```python
from build123d import *

# Parameters (mm, degrees)
SKETCH1_W           = 12.7
SKETCH1_H           = 12.7
BOSS_EXTRUDE1_DEPTH = 1.6002
SKETCH2_W           = 12.7
SKETCH2_H           = 11.7602
BOSS_EXTRUDE2_DEPTH = 1.6002
SKETCH3_W           = 12.7
SKETCH3_H           = 1.6002
BOSS_EXTRUDE3_DEPTH = 9.525
SKETCH4_R           = 2.5527
CUT_EXTRUDE1_DEPTH  = 22.187985158
FILLET1_R           = 0.762


with BuildPart() as part:
    # Sketch1 → Boss-Extrude1 (new body)
    with BuildSketch(Plane(origin=(0, 0, 0), x_dir=(1, 0, 0), z_dir=(0, 1, 0))):
        Rectangle(SKETCH1_W, SKETCH1_H)
    extrude(amount=BOSS_EXTRUDE1_DEPTH)

    # Sketch2 → Boss-Extrude2 (add)
    with BuildSketch(Plane(origin=(6.35, 0, 0), x_dir=(0, 0, -1), z_dir=(1, 0, 0))):
        with Locations((0, -4.2799)):
            Rectangle(SKETCH2_W, SKETCH2_H)
    boss_extrude2 = extrude(amount=BOSS_EXTRUDE2_DEPTH)

    # Sketch3 → Boss-Extrude3 (add)
    with BuildSketch(Plane(origin=(7.9502, 0, 0), x_dir=(0, 0, -1), z_dir=(1, 0, 0))):
        with Locations((0, -9.3599)):
            Rectangle(SKETCH3_W, SKETCH3_H)
    boss_extrude3 = extrude(amount=BOSS_EXTRUDE3_DEPTH)

    # Sketch4 → Cut-Extrude1 (cut, through all)
    with BuildSketch(Plane(origin=(0, -8.5598, 0), x_dir=(1, 0, 0), z_dir=(0, 1, 0))):
        with Locations(Location((12.7127, 0, 0), (0, 0, 270))):
            Circle(SKETCH4_R)
    cut_extrude1 = extrude(amount=-CUT_EXTRUDE1_DEPTH, mode=Mode.SUBTRACT)

    # Mirror2: Boss-Extrude2, Boss-Extrude3, Cut-Extrude1 across plane
    add(boss_extrude2.mirror(Plane(origin=(0, 0, 0), x_dir=(0, 0, 1), z_dir=(1, 0, 0))))
    add(boss_extrude3.mirror(Plane(origin=(0, 0, 0), x_dir=(0, 0, 1), z_dir=(1, 0, 0))))
    add(cut_extrude1.mirror(Plane(origin=(0, 0, 0), x_dir=(0, 0, 1), z_dir=(1, 0, 0))), mode=Mode.SUBTRACT)

    # Fillet1
    fillet1_edges = [part.edges().sort_by_distance(p)[0] for p in [
        (6.35, -10.16, 0),
        (-6.35, -10.16, 0),
        (6.35, 0, 0),
        (-6.35, 0, 0),
        (-7.9502, -8.5598, 0),
        (-7.9502, 1.6002, 0),
        (7.9502, 1.6002, 0),
        (7.9502, -8.5598, 0),
    ]]
    fillet(fillet1_edges, radius=FILLET1_R)


solid = part.part
```
Geometry check sheet. Reference: the model listing, model coordinates, mm. A direction names the side the tool comes from. Coordinates: 2 decimals unless noted, no trailing zeros. Loops run counter-clockwise (first coordinate to the right, second up) from the corner with the lowest first, then second, coordinate; pieces in that order, holes last.
Item 1: Access from +Z, -Z, +X, -X, +Y, -Y to the whole of each face (thin tool, end or side, straight path). Record for faces 5 (the face through (-7.95, -3, 0)), 6 (the face through (6.35, -5, 0)), 7 (the face through (7.95, -3, 0)).
Item 2: Sectioned sample at C-C, the plane x = -14. Record the boundary of the cut face in (y, z), then the cut area to 3 significant figures.
Item 3: Sectioned sample at B-B, the plane y = -5.75. Record the boundary of the cut face in (x, z).
Item 4: Sectioned sample at A-A, the plane z = 0. Record the boundary of the cut face in (x, y).
Item 5: Thickness scan on line 1 (X direction, y = -9.2, z = 0); line 2 (X direction, y = -9.25, z = 4); line 3 (X direction, y = -3.25, z = -5). Record the ranges inside material, lowest first.
Item 6: Release check for a two-part mould opening along Z. For faces 1 (the face through (15, -8.56, 2)), 2 (the face through (15.244, -9.349, -0.332)), 3 (the face through (-15.244, -9.349, -0.332)), 4 (the face through (0.1, 0.5, -6.35)) record: released by +Z, released by -Z, zero draft, split by the parting line, or undercut.
Item 7: Go/stop test with flat-tipped pins: pin 1 Ø4 at (x, z) = (12.71, 0) entering from -Y; pin 2 Ø1.5 at (x, z) = (1, 2) entering from -Y; pin 3 Ø7 at (y, z) = (-4, -0.5) entering from -X; pin 4 Ø6 at (x, z) = (9, 4.5) entering from +Y. Record where each tip stops, or that it passes through.
Item 8: Sectioned sample at D-D, the plane z = -2. Record the boundary of the cut face in (x, y).
Check result:
1. face 5: +Z, -Z, -X, +Y
1. face 6: +Z, -Z, -Y
1. face 7: +Z, -Z, +X, +Y
2. outline: (-10.16, -6.35) - (-8.56, -6.35) - (-8.56, -2.2) - (-10.16, -2.2) - close; (-10.16, 2.2) - (-8.56, 2.2) - (-8.56, 6.35) - (-10.16, 6.35) - close
2. area: 13.3 mm2
3. outline: (-7.95, -6.35) - (-6.35, -6.35) - (-6.35, 6.35) - (-7.95, 6.35) - close; (6.35, -6.35) - (7.95, -6.35) - (7.95, 6.35) - (6.35, 6.35) - close
4. outline: (-17.48, -10.16) - (-15.27, -10.16) - (-15.27, -8.56) - (-17.48, -8.56) - close; (-10.16, -10.16) - (-7.11, -10.16) arc R0.76 ccw to (-6.35, -9.4) - (-6.35, -0.76) arc R0.76 cw to (-5.59, 0) - (5.59, 0) arc R0.76 cw to (6.35, -0.76) - (6.35, -9.4) arc R0.76 ccw to (7.11, -10.16) - (10.16, -10.16) - (10.16, -8.56) - (8.71, -8.56) arc R0.76 cw to (7.95, -7.8) - (7.95, 0.84) arc R0.76 ccw to (7.19, 1.6) - (-7.19, 1.6) arc R0.76 ccw to (-7.95, 0.84) - (-7.95, -7.8) arc R0.76 cw to (-8.71, -8.56) - (-10.16, -8.56) - close; (15.27, -10.16) - (17.48, -10.16) - (17.48, -8.56) - (15.27, -8.56) - close
5. line 1: x = -17.48 to -15.27, -10.16 to -6.35, 6.35 to 10.16, 15.27 to 17.48
5. line 2: x = -17.48 to -6.35, 6.35 to 17.48
5. line 3: x = -7.95 to -6.35, 6.35 to 7.95
6. face 1: zero draft
6. face 2: undercut
6. face 3: undercut
6. face 4: released by -Z
7. pin 1: passes through
7. pin 2: stops at y = 0
7. pin 3: stops at x = -7.95
7. pin 4: stops at y = 1.6
8. outline: (-17.48, -10.16) - (-14.3, -10.16) - (-14.3, -8.56) - (-17.48, -8.56) - close; (-11.13, -10.16) - (-7.11, -10.16) arc R0.76 ccw to (-6.35, -9.4) - (-6.35, -0.76) arc R0.76 cw to (-5.59, 0) - (5.59, 0) arc R0.76 cw to (6.35, -0.76) - (6.35, -9.4) arc R0.76 ccw to (7.11, -10.16) - (11.13, -10.16) - (11.13, -8.56) - (8.71, -8.56) arc R0.76 cw to (7.95, -7.8) - (7.95, 0.84) arc R0.76 ccw to (7.19, 1.6) - (-7.19, 1.6) arc R0.76 ccw to (-7.95, 0.84) - (-7.95, -7.8) arc R0.76 cw to (-8.71, -8.56) - (-11.13, -8.56) - close; (14.3, -10.16) - (17.48, -10.16) - (17.48, -8.56) - (14.3, -8.56) - close
